```python
from build123d import *

# Parameters (mm, degrees)
F0_W     = 35.56
F0_H     = 35.56
F1_DEPTH = 5.08
F2_W     = 19.812
F2_H     = 4.572
F3_DEPTH = 2.54
F4_W     = 19.812
F4_H     = 4.572
F5_DEPTH = 2.54
F6_W     = 20.32
F6_H     = 5.08
F7_DEPTH = 2.54
F8_W     = 20.32
F8_H     = 5.08
F9_DEPTH = 2.54


with BuildPart() as f1:
    # F0 (on Top) → F1 (new body, symmetric)
    with BuildSketch(Plane.XY):
        Rectangle(F0_W, F0_H)
        Polygon((-6.3637803819, 12.4850260417), (-1.1437717014, 2.1166666667), (4.1093098958, 12.4850260417), (9.8639973958, 12.4850260417), (1.5075737847, -2.8993923611), (1.5075737847, -12.7), (-3.7951171875, -12.7), (-3.7951171875, -3.0702690972), (-12.1515407986, 12.4850260417), align=None, mode=Mode.SUBTRACT)
    extrude(amount=F1_DEPTH, both=True)

    # F2 (on face) → F3 (join)
    with BuildSketch(Plane(origin=(0, 17.78, 0), x_dir=(-1, 0, 0), z_dir=(0, 1, 0))):
        Rectangle(F2_W, F2_H)
    extrude(amount=F3_DEPTH)

    # F4 (on face) → F5 (join)
    with BuildSketch(Plane(origin=(-17.78, 0, 0), x_dir=(0, -1, 0), z_dir=(-1, 0, 0))):
        Rectangle(F4_W, F4_H)
    extrude(amount=F5_DEPTH)

    # F6 (on face) → F7 (cut)
    with BuildSketch(Plane.XZ.offset(17.78)):
        Rectangle(F6_W, F6_H)
    extrude(amount=-F7_DEPTH, mode=Mode.SUBTRACT)

    # F8 (on face) → F9 (cut)
    with BuildSketch(Plane.YZ.offset(17.78)):
        Rectangle(F8_W, F8_H)
    extrude(amount=-F9_DEPTH, mode=Mode.SUBTRACT)


solid = f1.part
```
Source: CAD feature listing. Evaluate the final solid. Frame: model axes, mm. A direction names the side the tool comes from. Round coordinates to 2 decimals unless told otherwise and drop trailing zeros. Order: outer loops, then holes, each group sorted by start corner. A loop starts at its lowest first (then second) coordinate and runs counter-clockwise, first axis right, second up. Notation, with made-up numbers: (-28, 60.5) -> (27, 60.5) arc R21 cw to (27, 98.5) -> close; hole circle Ø9 at (-6, 9). An arc over 180 degrees is marked (long way). Use CSV: the item, a comma, the result in double quotes.
(1) Section B-B on y = -4. Return the cut outline in (x, z), and give its area (3 significant figures).
Report:
outline,"(-20.32, -2.29) -> (-17.78, -2.29) -> (-17.78, -5.08) -> (-3.8, -5.08) -> (-3.8, 5.08) -> (-17.78, 5.08) -> (-17.78, 2.29) -> (-20.32, 2.29) -> close; (1.51, -5.08) -> (17.78, -5.08) -> (17.78, -2.54) -> (15.24, -2.54) -> (15.24, 2.54) -> (17.78, 2.54) -> (17.78, 5.08) -> (1.51, 5.08) -> close"
area,"306 mm^2"
(2) Section A-A on z = -3.25. Return the cut outline in (x, y), and give its area (3 significant figures).
Report:
outline,"(-17.78, -17.78) -> (17.78, -17.78) -> (17.78, 17.78) -> (-17.78, 17.78) -> close; hole (-12.15, 12.49) -> (-3.8, -3.07) -> (-3.8, -12.7) -> (1.51, -12.7) -> (1.51, -2.9) -> (9.86, 12.49) -> (4.11, 12.49) -> (-1.14, 2.12) -> (-6.36, 12.49) -> close"
area,"1,060 mm^2"
(3) Section C-C on x = -11.5. Return the cut outline in (y, z).
Report:
outline,"(-17.78, -5.08) -> (11.27, -5.08) -> (11.27, 5.08) -> (-17.78, 5.08) -> close; (12.49, -5.08) -> (17.78, -5.08) -> (17.78, 5.08) -> (12.49, 5.08) -> close"
(4) Pull-direction query (Z, two-part tool) for faces 4 (the face through (17, -10.16, 0)), 5 (the face through (0, 19, 2.286)), 6 (the face through (-9.906, 19, 0)); classes: +Z half, -Z half, draft (parallel to the pull), parting line (faces both ways), or undercut.
Report:
face 4,"undercut"
face 5,"+Z half"
face 6,"draft"
(5) Ray query, L1, parallel to X at y = -16, z = -1; L2, parallel to X at y = 9.5, z = -3; L3, parallel to X at y = -11, z = -2.25. Return the intervals inside material, ascending.
Report:
L1,"-17.78 to -10.16, 10.16 to 17.78"
L2,"-17.78 to -10.55, -4.86 to 2.6, 8.24 to 17.78"
L3,"-17.78 to -3.8, 1.51 to 17.78"
(6) Access query for faces 1 (the face through (-19, 0, 2.286)), 2 (the face through (17, 0, 2.54)), 3 (the face through (7, 12.485, 0)). Directions: +Z, -Z, +X, -X, +Y, -Y. A direction counts if a zero-diameter tool reaches every point of the face in a straight line with its end or side. Return the directions, or none.
Report:
face 1,"+Z, -X, +Y, -Y"
face 2,"+X"
face 3,"+Z, -Z"
(7) First-contact query: pin 1 Ø5 at (x, z) = (5, 1) entering from -Y; pin 2 Ø3 at (x, z) = (-19.5, 0.5) entering from +Y; pin 3 Ø3 at (x, z) = (17, -1) entering from +Y; pin 4 Ø3 at (x, z) = (-8.5, -1) entering from -Y. Flat tips, straight axial feed; report the tip coordinate or a pass-through.
Report:
pin 1,"y = -17.78"
pin 2,"y = 9.91"
pin 3,"y = 17.78"
pin 4,"y = -15.24"
